from build123d import *

# Parameters (mm, degrees)
SKETCH1_R                                 = 9.525
BOSS_EXTRUDE1_DEPTH                       = 19.05
SKETCH2_OUTSIDE_W                         = 62.28
SKETCH2_OUTSIDE_H                         = 106.73
CUT_EXTRUDE1_DEPTH                        = 31.75
FILLET1_R                                 = 3.175
FILLET2_R                                 = 25.4
CBORE_FOR_5_16_HEX_CAP_SCREW1_D           = 8.4328
CBORE_FOR_5_16_HEX_CAP_SCREW1_DEPTH       = 15.875
CBORE_FOR_5_16_HEX_CAP_SCREW1_CBORE_D     = 20.6375
CBORE_FOR_5_16_HEX_CAP_SCREW1_CBORE_DEPTH = 5.969


with BuildPart() as part:
    # Sketch1 → Boss-Extrude1 (new body, symmetric)
    with BuildSketch(Plane.XY):
        with BuildLine():
            Line((17.184764726, 8.221092465), (31.75, -22.225))
            Line((31.75, -22.225), (31.75, -63.5))
            Line((31.75, -63.5), (15.875, -63.5))
            Line((15.875, -63.5), (15.875, -22.225))
            Line((15.875, -22.225), (-15.875, -22.225))
            Line((-15.875, -22.225), (-15.875, -63.5))
            Line((-15.875, -63.5), (-31.75, -63.5))
            Line((-31.75, -63.5), (-31.75, -22.225))
            Line((-31.75, -22.225), (-17.184764726, 8.221092465))
            ThreePointArc((-17.184764726, 8.221092465), (0, 19.05), (17.184764726, 8.221092465))
        make_face()
        Circle(SKETCH1_R, mode=Mode.SUBTRACT)
    extrude(amount=BOSS_EXTRUDE1_DEPTH, both=True)

    # Sketch2 outside → Cut-Extrude1 (cut, symmetric)
    with BuildSketch(Plane(origin=(0, 0, 0), x_dir=(0, 0, -1), z_dir=(1, 0, 0))):
        with Locations((0, -22.225)):
            Rectangle(SKETCH2_OUTSIDE_W, SKETCH2_OUTSIDE_H)
        with BuildLine():
            Line((18.897197735, -42.042009604), (11.1125, 19.05))
            Line((11.1125, 19.05), (-11.1125, 19.05))
            Line((-11.1125, 19.05), (-18.897197735, -42.042009604))
            ThreePointArc((-18.897197735, -42.042009604), (0, -63.5), (18.897197735, -42.042009604))
        make_face(mode=Mode.SUBTRACT)
    extrude(amount=CUT_EXTRUDE1_DEPTH, both=True, mode=Mode.SUBTRACT)

    # Fillet1
    fillet1_edges = [part.edges().sort_by_distance(p)[0] for p in [
        (15.875, -22.225, 0),
        (-15.875, -22.225, 0),
    ]]
    fillet(fillet1_edges, radius=FILLET1_R)

    # Fillet2
    fillet2_edges = [part.edges().sort_by_distance(p)[0] for p in [
        (31.75, -22.225, 0),
        (-31.75, -22.225, 0),
    ]]
    fillet(fillet2_edges, radius=FILLET2_R)

    # CBORE for 5/16 Hex Cap Screw1
    with Locations(Plane(origin=(-15.875, 0, 0), x_dir=(0, 0, -1), z_dir=(1, 0, 0))):
        with Locations((0, -44.45)):
            cbore_for_5_16_hex_cap_screw1 = CounterBoreHole(CBORE_FOR_5_16_HEX_CAP_SCREW1_D / 2, CBORE_FOR_5_16_HEX_CAP_SCREW1_CBORE_D / 2, CBORE_FOR_5_16_HEX_CAP_SCREW1_CBORE_DEPTH, depth=CBORE_FOR_5_16_HEX_CAP_SCREW1_DEPTH)

    # Mirror1: CBORE for 5/16 Hex Cap Screw1 across plane
    add(cbore_for_5_16_hex_cap_screw1.mirror(Plane(origin=(0, 0, 0), x_dir=(0, 0, 1), z_dir=(1, 0, 0))), mode=Mode.SUBTRACT)


solid = part.part
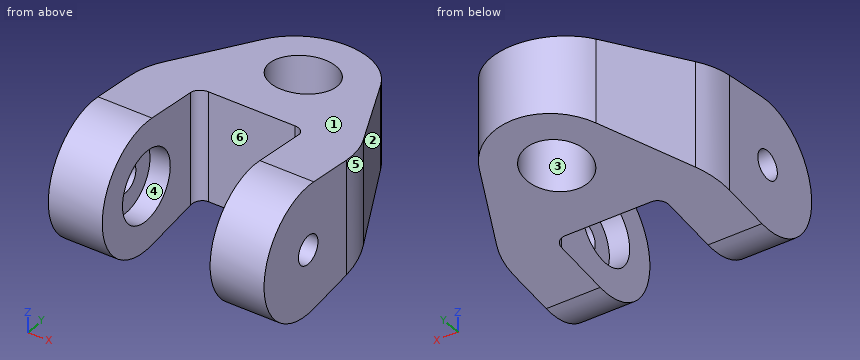
Can you work these out from the model? Positions are in its coordinate system, mm. Face numbers are marked on the shaded views. A direction names the side the tool comes from. Coordinates: 2 decimals unless noted, no trailing zeros. Write each loop counter-clockwise with the first axis right and the second up, starting at its lowest first coordinate (ties: lowest second). Pieces come first, ordered by that corner, then holes. Notation, with made-up numbers: (25.5, 73) -> (78.5, 73) arc R18 ccw to (78.5, 94) -> close; hole circle Ø8 at (40, 37). An arc over 180 degrees is marked (long way). Answer as CSV lines item,"result".
1) If we section it at D-D on z = -9: Please give me the cut outline in (x, y) (3 decimals).
Check result:
outline,"(-31.75, -61.24) -> (-15.875, -61.24) -> (-15.875, -49.497) -> (-21.844, -49.497) -> (-21.844, -39.403) -> (-15.875, -39.403) -> (-15.875, -25.4) arc R3.175 cw to (-12.7, -22.225) -> (12.7, -22.225) arc R3.175 cw to (15.875, -25.4) -> (15.875, -39.403) -> (21.844, -39.403) -> (21.844, -49.497) -> (15.875, -49.497) -> (15.875, -61.24) -> (31.75, -61.24) -> (31.75, -27.988) arc R25.4 ccw to (29.263, -17.026) -> (17.185, 8.221) arc R19.05 ccw to (-17.185, 8.221) -> (-29.263, -17.026) arc R25.4 ccw to (-31.75, -27.988) -> close; hole circle Ø19.05 at (0, 0)"
2) If we mould it in two halves opening along X, with no side actions, what happens to the marked faces 1, 2 and 3? For each: +X half, -X half, draft (parallel to the pull), parting line (faces both ways), or undercut.
Check result:
face 1,"draft"
face 2,"+X half"
face 3,"undercut"
3) If we section it at A-A on z = 0: Count the separate pieces of the cut face and the enclosed holes in it, then the cut area to 3 significant figures.
Check result:
separate pieces,"3"
enclosed holes,"1"
area,"2,370 mm²"
4) Will these pins go through, and if not, where does the flat tip stop? P1, Ø22, axis at x = 0, y = 0, coming from the +Z side; P2, Ø8, axis at x = 2.5, y = -16, coming from the -Z side; P3, Ø6, axis at x = 13.5, y = -4, coming from the -Z side.
Check result:
P1,"z = 14.94"
P2,"z = -16.09"
P3,"z = -14.43"
5) If we section it at B-B on y = -44.45: Please give me the cut outline in (x, z) (3 decimals), then the cut area to 3 significant figures.
Check result:
outline,"(-31.75, -19.05) -> (-15.875, -19.05) -> (-15.875, -10.319) -> (-21.844, -10.319) -> (-21.844, -4.216) -> (-31.75, -4.216) -> close; (-31.75, 4.216) -> (-21.844, 4.216) -> (-21.844, 10.319) -> (-15.875, 10.319) -> (-15.875, 19.05) -> (-31.75, 19.05) -> close; (15.875, -19.05) -> (31.75, -19.05) -> (31.75, -4.216) -> (21.844, -4.216) -> (21.844, -10.319) -> (15.875, -10.319) -> close; (15.875, 10.319) -> (21.844, 10.319) -> (21.844, 4.216) -> (31.75, 4.216) -> (31.75, 19.05) -> (15.875, 19.05) -> close"
area,"796 mm²"
6) On a 3-axis mill with a long thin cutter (end or side, diameter ignored), from which of +Z, -Z, +X, -X, +Y, -Y can I reach the whole of each face in a straight line? I mean the marked faces 4, 5 and 6. Say none if no direction works.
Check result:
face 4,"none"
face 5,"+Z, -Z, +X, +Y"
face 6,"+Z, -Z, -Y"
7) If I drill on line 1 (Z direction, x = 18.1, y = -44.45); line 2 (Y direction, x = 0, z = 3) (3 decimals); line 3 (X direction, y = -54.5, z = 13) (3 decimals), over which ranges is the centre line in solid material (lowest first)? Write a range as from..to.
Check result:
line 1,"-19.05..-10.32, 10.32..19.05"
line 2,"-22.225..-9.525, 9.525..19.05"
line 3,"-31.75..-15.875, 15.875..31.75"
8) If we section it at C-C on x = 4.5: Please give me the cut outline in (y, z) (3 decimals), then the cut area to 3 significant figures.
Check result:
outline,"(-22.225, -16.372) -> (-8.395, -14.61) -> (-8.395, 14.61) -> (-22.225, 16.372) -> close; (8.395, -12.47) -> (18.511, -11.181) -> (18.511, 11.181) -> (8.395, 12.47) -> close"
area,"668 mm²"
